from build123d import *

# Parameters (mm, degrees)
F1_DEPTH = 60
F2_DEPTH = 42
F3_DEPTH = 42


with BuildPart() as f1:
    # F0 (on Front) → F1 (new body)
    with BuildSketch(Plane.XZ):
        with BuildLine():
            ThreePointArc((-9, 1.369445934), (-4.5828518842, 0.1402203037), (0, 0))
            Line((0, 0), (0, 3))
            Line((0, 3), (-9, 3))
            ThreePointArc((-9, 3), (-9.5190631598, 2.184722967), (-9, 1.369445934))
        make_face()
    extrude(amount=F1_DEPTH)

    # F2 (add): a face of the model
    f2_faces = [f1.faces().sort_by_distance(p)[0] for p in [
        (-4.2472237482, -60, 1.6364055224),
    ]]
    extrude(f2_faces, amount=-F2_DEPTH)

    # F3 (cut): a face of the model
    f3_faces = [f1.faces().sort_by_distance(p)[0] for p in [
        (-4.2472237482, -60, 1.6364055224),
    ]]
    extrude(f3_faces, amount=-F3_DEPTH, mode=Mode.SUBTRACT)


solid = f1.part
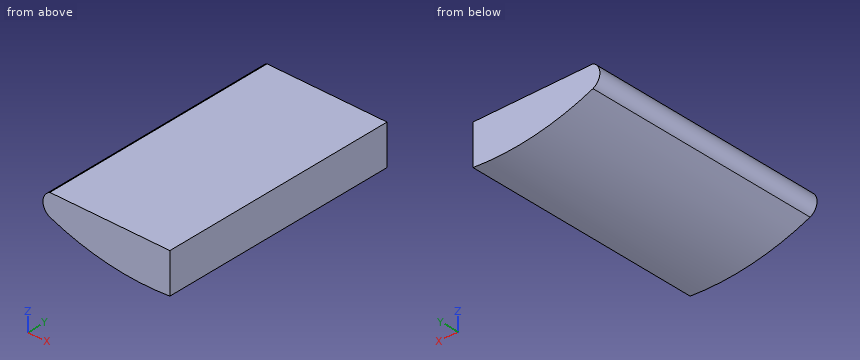
Check sheet for the modelled part. Datum: model origin and axes. Units: mm. Round coordinates to 2 decimals unless told otherwise and drop trailing zeros. Write each loop counter-clockwise with the first axis right and the second up, starting at its lowest first coordinate (ties: lowest second). Pieces come first, ordered by that corner, then holes. Notation, with made-up numbers: (-34, 68) - (-23, 68) arc R18 ccw to (-23, 95) - close; hole circle Ø10 at (-38.75, 49). An arc over 180 degrees is marked (long way). Return JSON: item names as keys, results as strings.
Q1. Depth check by flat-ended pin: P1, Ø1.5, axis at x = -7, y = -6, coming from the -Z side; P2, Ø3, axis at x = -2, y = -12, coming from the -Z side. Enter the tip coordinate at first touch or a pass-through.
Returned:
{"P1": "stops at z = 0.47", "P2": "stops at z = -0.08"}
Q2. Cross-section at B-B (x = -8.25). Record the boundary of the cut face in (y, z), then the cut area to 3 significant figures.
Returned:
{"outline": "(-18, 1.08) - (0, 1.08) - (0, 3) - (-18, 3) - close", "area": "34.6 mm²"}
Q3. Scan lines: L1, parallel to Z at x = -1.75, y = -3; L2, parallel to Z at x = -5.25, y = -4.25; L3, parallel to X at y = -13, z = 2.6. Record each from-to range of solid material in increasing order. Write a range as from..to.
Returned:
{"L1": "z = -0.08..3", "L2": "z = 0.25..3", "L3": "x = -9.42..0"}
Q4. Cross-section at A-A (y = -3). Record the boundary of the cut face in (x, z), then the cut area to 3 significant figures.
Returned:
{"outline": "(-9, 1.37) arc R19.08 ccw to (0, 0) - (0, 3) - (-9, 3) arc R0.9 ccw to start", "area": "24.8 mm²"}
